from build123d import *

# Parameters (mm, degrees)
BOSS_EXTRUDE1_START = 4
SKETCH2_R           = 3.9
BOSS_EXTRUDE1_DEPTH = 2
SKETCH3_W           = 3
SKETCH3_H           = 0.4
BOSS_EXTRUDE2_DEPTH = 7
CIRPATTERN1_COUNT   = 3
CIRPATTERN1_ANGLE   = 180


with BuildPart() as part:
    # Sketch1 → Revolve1 (revolve)
    with BuildSketch(Plane(origin=(0, 0, 0), x_dir=(0, 0, -1), z_dir=(1, 0, 0))):
        with BuildLine():
            Line((-3.9, 13.7), (-3.9, 8))
            Line((-3.9, 8), (-5.5, 8))
            Line((-5.5, 8), (-5.5, 5))
            Line((-5.5, 5), (-4, 5))
            Line((-4, 5), (-4, 0))
            Line((-4, 0), (0, 0))
            Line((0, 0), (0, 12.2))
            ThreePointArc((0, 12.2), (-0.883883476, 11.833883476), (-1.25, 10.95))
            Line((-1.25, 10.95), (-1.25, 6.7))
            Line((-1.25, 6.7), (-2.9, 6.7))
            Line((-2.9, 6.7), (-2.9, 12.7))
            Line((-2.9, 12.7), (-3.9, 13.7))
        make_face()
    revolve(axis=Axis((0, 12.2, 0), (0, -1, 0)))

    # Sketch2 → Boss-Extrude1 (add)
    with BuildSketch(Plane(origin=(0, 8, 0), x_dir=(1, 0, 0), z_dir=(0, 1, 0)).offset(BOSS_EXTRUDE1_START)):
        Polygon((5.3, 3.059956427), (0, 6.119912853), (-5.3, 3.059956427), (-5.3, -3.059956427), (0, -6.119912853), (5.3, -3.059956427), align=None)
        Circle(SKETCH2_R, mode=Mode.SUBTRACT)
    extrude(amount=BOSS_EXTRUDE1_DEPTH)

    # Sketch3 → Boss-Extrude2 (add)
    with BuildSketch(Plane.XZ):
        with Locations((0, 3.508099244)):
            Rectangle(SKETCH3_W, SKETCH3_H)
    boss_extrude2 = extrude(amount=BOSS_EXTRUDE2_DEPTH)

    # CirPattern1: Boss-Extrude2 ×3 about axis
    cirpattern1_axis = Axis((0, 0, 0), (0, 1, 0))
    for i in range(1, CIRPATTERN1_COUNT):
        add(boss_extrude2.rotate(cirpattern1_axis, i * CIRPATTERN1_ANGLE / (CIRPATTERN1_COUNT - 1)))


solid = part.part
The model under review builds one solid part; all positions refer to its coordinate system, in mm. A direction names the side the tool comes from. Round coordinates to 2 decimals unless told otherwise and drop trailing zeros. Loops run counter-clockwise (first coordinate to the right, second up) from the corner with the lowest first, then second, coordinate; pieces in that order, holes last. Notation, with made-up numbers: (-7.75, 76.25) -> (19.25, 76.25) arc R14 ccw to (19.25, 91.25) -> close; hole circle Ø11 at (40, 41.25). An arc over 180 degrees is marked (long way). Write item = value, one per line. Start each with the question number.
Item 1: Insertion check: pin 1 (4 mm diameter, centred on y = 1.5, z = 2.5, fed in from -X); pin 2 (1.6 mm diameter, centred on y = 13.5, z = -1, fed in from -X); pin 3 (3.5 mm diameter, centred on x = -0.5, y = -4.5, fed in from -Z); pin 4 (1 mm diameter, centred on x = 0.5, z = -3, fed in from -Y). Each pin has a flat end and moves straight along its axis. Give the tip position at first contact, or say it passes through.
Item 2: Mouldability with a two-part tool opening along Y and no side actions: class faces 5 (the flat face through (1, 6.7, -1)), 6 (the cylindrical face through (1.22, 8.8, -0.27)), 7 (the cylindrical face through (-1.17, 9.97, 3.72)), 8 (the flat face through (2, 5, -4)) as released by +Y, released by -Y, zero draft, split by the parting line, or undercut.
Item 3: Take a section at B-B on y = 8.75. Give the boundary of the cut face in (x, z).
Item 4: Take a section at A-A on y = -4.5. Give the boundary of the cut face in (x, z), plus the area to 3 significant figures.
Item 5: Take a section at D-D on y = 4.75. Give the boundary of the cut face in (x, z), plus the area to 3 significant figures.
Item 6: To check wall thickness, follow L1, parallel to Z at x = 0, y = 10.05; L2, parallel to Y at x = -5, z = -1.25. State the ranges of each line that lie inside material, in increasing order.
Item 7: For faces 1 (the flat face through (0, -3, 3.308)), 2 (the flat face through (2.613, 12.986, 4.611)), 3 (the cylindrical face through (-0.1, 9.7, -2.9)), 4 (the cylindrical face through (5.37, 6.48, -1.19)), list the 3-axis set-ups (+Z, -Z, +X, -X, +Y, -Y) from which the entire face can be reached by the end or side of a thin tool; tool diameter is ignored.
Result:
q1.pin_1 = -3.97
q1.pin_2 = -5.3
q1.pin_3 = -3.71
q1.pin_4 = -7
q2.face_5 = released by +Y
q2.face_6 = zero draft
q2.face_7 = undercut
q2.face_8 = released by -Y
q3.outline = circle Ø7.8 at (0, 0); circle Ø2.5 at (0, 0); hole circle Ø5.8 at (0, 0)
q4.outline = (-1.5, -3.71) -> (1.5, -3.71) -> (1.5, -3.31) -> (-1.5, -3.31) -> close; (-1.5, 3.31) -> (1.5, 3.31) -> (1.5, 3.71) -> (-1.5, 3.71) -> close; (3.31, -1.5) -> (3.71, -1.5) -> (3.71, 1.5) -> (3.31, 1.5) -> close
q4.area = 3.60 mm²
q5.outline = circle Ø8 at (0, 0)
q5.area = 50.3 mm²
q6.L1 = -3.9 to -2.9, -1.25 to 1.25, 2.9 to 3.9
q6.L2 = 5 to 8, 12 to 14
q7.face_1 = +X, -X, -Y
q7.face_2 = +Z, +X, +Y
q7.face_3 = +Y
q7.face_4 = -Y
